```python
from build123d import *

# Parameters (mm, degrees)
BOSS_EXTRUDE1_DEPTH = 30
BOSS_EXTRUDE2_DEPTH = 3
SKETCH7_R           = 3.4
SKETCH7_W           = 26.6
SKETCH7_H           = 15.7
SKETCH7_W_2         = 20.5
SKETCH7_H_2         = 24
CUT_EXTRUDE1_DEPTH  = 3
SKETCH8_W           = 10
SKETCH8_H           = 10
BOSS_EXTRUDE3_DEPTH = 27
SKETCH9_R           = 3
CUT_EXTRUDE2_DEPTH  = 20
SKETCH10_W          = 12.5
SKETCH10_H          = 18.5
CUT_EXTRUDE3_DEPTH  = 10
BOSS_EXTRUDE4_DEPTH = 1.5
SKETCH14_R          = 2
BOSS_EXTRUDE5_DEPTH = 5
BOSS_EXTRUDE6_START = 1
SKETCH15_R          = 3.4
BOSS_EXTRUDE6_DEPTH = 1


with BuildPart() as part:
    # Sketch1 → Boss-Extrude1 (new body)
    with BuildSketch(Plane.XY):
        with BuildLine():
            Line((-25, 75.5), (25, 75.5))
            ThreePointArc((25, 75.5), (34.192388155, 71.692388155), (38, 62.5))
            Line((38, 62.5), (38, -62.5))
            ThreePointArc((38, -62.5), (34.192388155, -71.692388155), (25, -75.5))
            Line((25, -75.5), (-25, -75.5))
            ThreePointArc((-25, -75.5), (-34.192388155, -71.692388155), (-38, -62.5))
            Line((-38, -62.5), (-38, 62.5))
            ThreePointArc((-38, 62.5), (-34.192388155, 71.692388155), (-25, 75.5))
        make_face()
        with BuildLine():
            Line((-25, 72.5), (25, 72.5))
            ThreePointArc((25, 72.5), (32.071067812, 69.571067812), (35, 62.5))
            Line((35, 62.5), (35, -62.5))
            ThreePointArc((35, -62.5), (32.071067812, -69.571067812), (25, -72.5))
            Line((25, -72.5), (-25, -72.5))
            ThreePointArc((-25, -72.5), (-32.071067812, -69.571067812), (-35, -62.5))
            Line((-35, -62.5), (-35, 62.5))
            ThreePointArc((-35, 62.5), (-32.071067812, 69.571067812), (-25, 72.5))
        make_face(mode=Mode.SUBTRACT)
    extrude(amount=-BOSS_EXTRUDE1_DEPTH)

    # Sketch6 → Boss-Extrude2 (add)
    with BuildSketch(Plane.XY):
        with BuildLine():
            Line((-23, -75.5), (23, -75.5))
            ThreePointArc((23, -75.5), (33.606601718, -71.106601718), (38, -60.5))
            Line((38, -60.5), (38, 60.5))
            ThreePointArc((38, 60.5), (33.606601718, 71.106601718), (23, 75.5))
            Line((23, 75.5), (-23, 75.5))
            ThreePointArc((-23, 75.5), (-33.606601718, 71.106601718), (-38, 60.5))
            Line((-38, 60.5), (-38, -60.5))
            ThreePointArc((-38, -60.5), (-33.606601718, -71.106601718), (-23, -75.5))
        make_face()
    extrude(amount=-BOSS_EXTRUDE2_DEPTH)

    # Sketch7 → Cut-Extrude1 (cut)
    with BuildSketch(Plane.XY):
        with Locations((0, -2)):
            Circle(SKETCH7_R)
        with Locations((0, 42.65)):
            Rectangle(SKETCH7_W, SKETCH7_H)
        with Locations((0, -50)):
            Rectangle(SKETCH7_W_2, SKETCH7_H_2)
    extrude(amount=-CUT_EXTRUDE1_DEPTH, mode=Mode.SUBTRACT)

    # Sketch8 → Boss-Extrude3 (add)
    with BuildSketch(Plane(origin=(0, 0, -3), x_dir=(-1, 0, 0), z_dir=(0, 0, -1))):
        with Locations((-25, 62.5)):
            Rectangle(SKETCH8_W, SKETCH8_H)
        with Locations((25, 62.5)):
            Rectangle(SKETCH8_W, SKETCH8_H)
        with Locations((25, -62.5)):
            Rectangle(SKETCH8_W, SKETCH8_H)
        with Locations((-25, -62.5)):
            Rectangle(SKETCH8_W, SKETCH8_H)
    extrude(amount=BOSS_EXTRUDE3_DEPTH)

    # Sketch9 → Cut-Extrude2 (cut)
    with BuildSketch(Plane(origin=(0, 0, -30), x_dir=(-1, 0, 0), z_dir=(0, 0, -1))):
        with Locations((-25, 62.5)):
            Circle(SKETCH9_R)
        with Locations((25, 62.5)):
            Circle(SKETCH9_R)
        with BuildLine():
            Line((-25.016555193, -65.499954321), (-24.983444807, -65.499954321))
            ThreePointArc((-24.983444807, -65.499954321), (-22.872834565, -64.615459102), (-22, -62.5))
            ThreePointArc((-22, -62.5), (-27.115459102, -60.372834565), (-25.016555193, -65.499954321))
        make_face()
        with Locations((25, -62.5)):
            Circle(SKETCH9_R)
    extrude(amount=-CUT_EXTRUDE2_DEPTH, mode=Mode.SUBTRACT)

    # Sketch10 → Cut-Extrude3 (cut)
    with BuildSketch(Plane.ZY.offset(38)):
        with Locations((-16.25, 34.886787821)):
            Rectangle(SKETCH10_W, SKETCH10_H)
    extrude(amount=-CUT_EXTRUDE3_DEPTH, mode=Mode.SUBTRACT)

    # Sketch12 → Boss-Extrude4 (add)
    with BuildSketch(Plane.XY):
        Polygon((5, -4.886751346), (5, 0.886751346), (0, 3.773502692), (-5, 0.886751346), (-5, -4.886751346), (0, -7.773502692), align=None)
    extrude(amount=BOSS_EXTRUDE4_DEPTH)

    # Sketch14 → Boss-Extrude5 (add)
    with BuildSketch(Plane.XY):
        with Locations((0, -2)):
            Circle(SKETCH14_R)
    extrude(amount=BOSS_EXTRUDE5_DEPTH)

    # Sketch15 → Boss-Extrude6 (add)
    with BuildSketch(Plane.XY.offset(5).offset(BOSS_EXTRUDE6_START)):
        with Locations((0, -2)):
            Circle(SKETCH15_R)
    extrude(amount=-BOSS_EXTRUDE6_DEPTH)


solid = part.part
```
Design review of the part built by this model. Coordinates are the model's own, in mm. A direction names the side the tool comes from. Round coordinates to 2 decimals unless told otherwise and drop trailing zeros. Write each loop counter-clockwise with the first axis right and the second up, starting at its lowest first coordinate (ties: lowest second). Pieces come first, ordered by that corner, then holes. Notation, with made-up numbers: (55, 17.5) -> (66, 17.5) arc R15 cw to (66, 33.5) -> close; hole circle Ø5 at (0, 11.5). An arc over 180 degrees is marked (long way). Answer in a Markdown table with one row per item.
Q1. Take a section at A-A, the plane y = -51. State the section outline as (x, z) points.
The answers:
| item | result |
|---|---|
| outline | (-38, -30) -> (-35, -30) -> (-35, -3) -> (-10.25, -3) -> (-10.25, 0) -> (-38, 0) -> close; (10.25, -3) -> (35, -3) -> (35, -30) -> (38, -30) -> (38, 0) -> (10.25, 0) -> close |
Q2. Take a section at C-C, the plane y = -2. State the section outline as (x, z) points, then the cut area to 3 significant figures.
The answers:
| item | result |
|---|---|
| outline | (-38, -30) -> (-35, -30) -> (-35, -3) -> (-3.4, -3) -> (-3.4, 0) -> (3.4, 0) -> (3.4, -3) -> (35, -3) -> (35, -30) -> (38, -30) -> (38, 0) -> (5, 0) -> (5, 1.5) -> (2, 1.5) -> (2, 5) -> (3.4, 5) -> (3.4, 6) -> (-3.4, 6) -> (-3.4, 5) -> (-2, 5) -> (-2, 1.5) -> (-5, 1.5) -> (-5, 0) -> (-38, 0) -> close |
| area | 405 mm² |
Q3. Clearance check with flat-ended pins moving along their axes: pin 1 Ø2.5 at (x, z) = (-36.5, -15.5) entering from -Y; pin 2 Ø5.5 at (x, y) = (0.5, -2) entering from -Z; pin 3 Ø2 at (x, z) = (27, -16) entering from +Y. State where each tip first meets the part, or that it passes through.
The answers:
| item | result |
|---|---|
| pin 1 | y = -70.5 |
| pin 2 | z = 0 |
| pin 3 | y = 75.46 |
Q4. Draft analysis for pull direction X (two halves, no side actions). For faces 1 (the face through (-34.091, -71.793, -14.79)), 2 (the face through (-10.25, -50, -1)), 3 (the face through (-23, -60, -30)), state which applies: +X half, -X half, draft (parallel to the pull), parting line (faces both ways), or undercut.
The answers:
| item | result |
|---|---|
| face 1 | -X half |
| face 2 | undercut |
| face 3 | draft |
Q5. To check wall thickness, follow L1, parallel to Y at x = -20.5, z = -18; L2, parallel to X at y = 58, z = -11; L3, parallel to Y at x = -12, z = -25. State the ranges of each line that lie inside material, in increasing order. Write a range as [from, to].
The answers:
| item | result |
|---|---|
| L1 | [-75.5, -72.5], [-67.5, -57.5], [57.5, 67.5], [72.5, 75.5] |
| L2 | [-38, -35], [-30, -20], [20, 30], [35, 38] |
| L3 | [-75.5, -72.5], [72.5, 75.5] |
Q6. For faces 4 (the face through (25, -67.5, -16)), 5 (the face through (0, -4.2, 5)), 6 (the face through (0, 50.5, -1)), 7 (the face through (-2.465, 2.35, 0.74)), 8 (the face through (37, 17, -30)), list the 3-axis set-ups (+Z, -Z, +X, -X, +Y, -Y) from which the entire face can be reached by the end or side of a thin tool; tool diameter is ignored.
The answers:
| item | result |
|---|---|
| face 4 | -Z |
| face 5 | none |
| face 6 | +Z, -Z |
| face 7 | +Z, -X, +Y |
| face 8 | -Z, +X, -X, +Y, -Y |
Q7. Take a section at B-B, the plane z = -16.5. Count the separate pieces of the cut face and the enclosed holes in it, then the cut area to 3 significant figures.
The answers:
| item | result |
|---|---|
| separate pieces | 5 |
| enclosed holes | 4 |
| area | 1,500 mm² |
